Design review of the part built by this model. Coordinates are the model's own, in mm. Face numbers are marked on the shaded views. A direction names the side the tool comes from. Round coordinates to 2 decimals unless told otherwise and drop trailing zeros. Loops run counter-clockwise (first coordinate to the right, second up) from the corner with the lowest first, then second, coordinate; pieces in that order, holes last. Notation, with made-up numbers: (-8, 5) - (33, 5) arc R23 ccw to (33, 37) - close; hole circle Ø10 at (80.5, 42). An arc over 180 degrees is marked (long way). Answer as CSV lines item,"result". Start each with the question number.
(1) Consider section D-D (x = 13). Give the boundary of the cut face in (y, z).
(2) Consider section B-B (z = 0). Give the boundary of the cut face in (x, y).
(3) Mouldability with a two-part tool opening along X and no side actions: class the marked faces 3, 4 and 5 as released by +X, released by -X, zero draft, split by the parting line, or undercut.
(4) Consider section A-A (y = 7). Give the boundary of the cut face in (x, z), and give its area (3 significant figures).
(5) For P1, Ø2.5, axis at x = 2, y = 8.5, coming from the +Z side; P2, Ø5, axis at x = 12, z = -9, coming from the +Y side; P3, Ø4, axis at y = 1, z = -11, coming from the -X side, all flat-tipped, find the tip position at first contact; note any pin that passes through.
(6) Wall thickness on L1, parallel to X at y = 6.55, z = 0; L2, parallel to X at y = 2.5, z = 0: over which ranges is each line inside the solid? List them lowest first.
(7) For the marked faces 1 and 2, list the 3-axis set-ups (+Z, -Z, +X, -X, +Y, -Y) from which the entire face can be reached by the end or side of a thin tool; tool diameter is ignored.
(8) Consider section C-C (x = 0). Give the boundary of the cut face in (y, z), and give its area (4 significant figures).
Autodesk Inventor part; units mm, degrees
ref_plane "Work Plane1" through (0, 4, 0) normal (0, 1, 0) x (1, 0, 0)
ref_plane "YZ Plane" through (0, 0, 0) normal (1, 0, 0) x (0, 1, 0)
ref_plane "XZ Plane" through (0, 0, 0) normal (0, 1, 0) x (-1, 0, 0)
sketch "Sketch1" plane through (0, 0, 0) normal (0, 1, 0) x (-1, 0, 0)
  circle A0 centre (0, 0) radius 23.75
  dimension "d0" = 47.5
extrude "Extrusion1" add sketch "Sketch1" along normal blind 5
sketch "Sketch2" plane through (0, 5, 0) normal (0, 1, 0) x (1, 0, 0)
  line L0 (-5, -5) -> (5, -5)
  line L1 (5, -5) -> (5, 5)
  line L2 (5, 5) -> (-5, 5)
  line L3 (-5, 5) -> (-5, -5)
  point P0 (0, 0)
  point P1 (-5, 0)
  point P2 (0, -5)
  dimension "d3" = 10
  dimension "d4" = 10
extrude "Extrusion2" add sketch "Sketch2" along normal blind 5
sketch "Sketch3" plane through (0, 10, 0) normal (0, 1, 0) x (1, 0, 0)
  circle A0 centre (0, 0) radius 2
  dimension "d7" = 4
sketch "Sketch4" plane through (0, 5, 0) normal (0, 1, 0) x (1, 0, 0)
  circle A0 centre (0, 0) radius 18.75
  circle A1 centre (0, 0) radius 23.75
  dimension "d8" = 5
extrude "Extrusion3" add sketch "Sketch4" along normal blind 3
extrude "Extrusion4" cut sketch "Sketch3" against normal up to next
ref_plane "Work Plane1" through (0, 4, 0) normal (0, 1, 0) x (1, 0, 0)
equation "\"d4\" = d3"
properties part number "wheel"
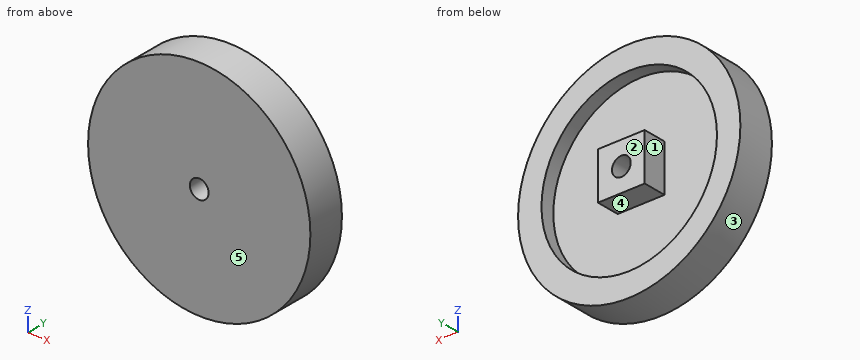
Determined:
1,outline,"(0, -19.88) - (8, -19.88) - (8, -13.51) - (5, -13.51) - (5, 13.51) - (8, 13.51) - (8, 19.88) - (0, 19.88) - close"
2,outline,"(-23.75, 0) - (-2, 0) - (-2, 10) - (-5, 10) - (-5, 5) - (-18.75, 5) - (-18.75, 8) - (-23.75, 8) - close; (2, 0) - (23.75, 0) - (23.75, 8) - (18.75, 8) - (18.75, 5) - (5, 5) - (5, 10) - (2, 10) - close"
3,face 3,"split by the parting line"
3,face 4,"undercut"
3,face 5,"zero draft"
4,outline,"circle Ø47.5 at (0, 0); (-5, -5) - (5, -5) - (5, 5) - (-5, 5) - close; hole circle Ø37.5 at (0, 0); hole circle Ø4 at (0, 0)"
4,area,"755 mm^2"
5,P1,"stops at z = 23.73"
5,P2,"stops at y = 5"
5,P3,"stops at x = -21.98"
6,L1,"x = -23.75 to -18.75, -5 to -2, 2 to 5, 18.75 to 23.75"
6,L2,"x = -23.75 to -2, 2 to 23.75"
7,face 1,"+Y"
7,face 2,"+Z, -Z, +X, -X, +Y"
8,outline,"(0, -23.75) - (8, -23.75) - (8, -18.75) - (5, -18.75) - (5, -5) - (10, -5) - (10, -2) - (0, -2) - close; (0, 2) - (10, 2) - (10, 5) - (5, 5) - (5, 18.75) - (8, 18.75) - (8, 23.75) - (0, 23.75) - close"
8,area,"277.5 mm^2"
